from build123d import *

# Parameters (mm, degrees)
SKETCH1_R               = 12.7
SKETCH1_R_2             = 6.35
BOSS_EXTRUDE1_DEPTH     = 7.62
CUT_EXTRUDE1_DEPTH      = 7.619999999999999
CUT_EXTRUDE1_DEPTH_BACK = 10.16
BOSS_EXTRUDE2_DEPTH     = 7.619999999999999
SKETCH5_R               = 1.905
SKETCH5_R_2             = 1.9050000000000018
CUT_EXTRUDE2_DEPTH      = 7.619999999999999


with BuildPart() as part:
    # Sketch1 → Boss-Extrude1 (new body)
    # profile 1 of 2: a face of its own
    with BuildSketch(Plane.XY):
        with Locations((-11.43, -2.615954225782393)):
            Circle(SKETCH1_R)
        with Locations((-11.43, -2.615954225782393)):
            Circle(SKETCH1_R_2, mode=Mode.SUBTRACT)
    # profile 2 of 2: a face of its own
    with BuildSketch(Plane.XY):
        Polygon((-8.7e-16, 22.784045774217606), (0, -28.01595422578239), (3.175, -28.01595422578239), (3.174999999999999, 22.784045774217606), align=None)
    extrude(amount=BOSS_EXTRUDE1_DEPTH)

    # Sketch3 → Cut-Extrude1 (cut, two sides: drawn at the far end of the back side and taken through both)
    with BuildSketch(Plane(origin=(5.715, 1e-16, 0), x_dir=(0, 0, -1), z_dir=(1, 2e-17, 0)).offset(-CUT_EXTRUDE1_DEPTH_BACK)):
        with BuildLine():
            ThreePointArc((-1.905, 15.116671425817602), (-2.4629615818396333, 16.46370984397798), (-3.810000000000017, 17.0216714258176))
            Line((-3.81, 17.0216714258176), (-3.81, 15.116671425817602))
            Line((-3.81, 15.116671425817602), (-3.81, 13.211671425817602))
            ThreePointArc((-3.8100000000000174, 13.211671425817602), (-2.4629615818396333, 13.769633007657223), (-1.905, 15.116671425817602))
        make_face()
        with BuildLine():
            Line((-3.81, 15.116671425817602), (-3.81, 17.0216714258176))
            ThreePointArc((-3.810000000000017, 17.0216714258176), (-5.715, 15.116671425817602), (-3.8100000000000174, 13.211671425817602))
            Line((-3.81, 13.211671425817602), (-3.81, 15.116671425817602))
        make_face()
        with BuildLine():
            ThreePointArc((-1.9049999999999947, -20.395954225782393), (-2.4629615818396298, -19.048915807622013), (-3.810000000000017, -18.490954225782392))
            Line((-3.81, -18.490954225782392), (-3.81, -20.395954225782393))
            Line((-3.81, -20.395954225782393), (-3.81, -22.300954225782395))
            ThreePointArc((-3.8100000000000156, -22.300954225782395), (-2.462961581839629, -21.742992643942774), (-1.9049999999999947, -20.395954225782393))
        make_face()
        with BuildLine():
            Line((-3.81, -20.395954225782393), (-3.81, -18.490954225782392))
            ThreePointArc((-3.810000000000017, -18.490954225782392), (-5.7149999999999945, -20.395954225782393), (-3.8100000000000156, -22.300954225782395))
            Line((-3.81, -22.300954225782395), (-3.81, -20.395954225782393))
        make_face()
    extrude(amount=CUT_EXTRUDE1_DEPTH + CUT_EXTRUDE1_DEPTH_BACK, mode=Mode.SUBTRACT)

    # Sketch4 → Boss-Extrude2 (add)
    with BuildSketch(Plane.XY.offset(7.62)):
        Polygon((3.174999999999999, 22.784045774217606), (5.715, 22.784045774217606), (5.715000000000006, -27.992122779019148), (3.174999999999999, -27.992122779019148), align=None)
    extrude(amount=-BOSS_EXTRUDE2_DEPTH)

    # Sketch5 → Cut-Extrude2 (cut)
    with BuildSketch(Plane(origin=(5.7150000000000025, 6.8e-16, 0), x_dir=(0, 0, -1), z_dir=(1, 1.2e-16, 0))):
        with Locations(Location((-3.81, 15.116671425817602, 0), (0, 0, 270))):
            Circle(SKETCH5_R)
        with Locations(Location((-3.8099999999999947, -20.395954225782393, 0), (0, 0, 270))):
            Circle(SKETCH5_R_2)
    extrude(amount=-CUT_EXTRUDE2_DEPTH, mode=Mode.SUBTRACT)


solid = part.part
The model under review builds one solid part; all positions refer to its coordinate system, in mm. A direction names the side the tool comes from. Give positions to 0.01 mm unless a question says otherwise; leave off trailing zeros. Loops run counter-clockwise (first coordinate to the right, second up) from the corner with the lowest first, then second, coordinate; pieces in that order, holes last. Notation, with made-up numbers: (40, 29.25) -> (73, 29.25) arc R20 ccw to (73, 64.25) -> close; hole circle Ø6 at (-7, 13). An arc over 180 degrees is marked (long way). Put each result on its own line as item: value. Start each with the question number.
1. We need section C-C on y = 16. State the section outline as (x, z) points (3 decimals).
2. We need section B-B on z = 4.5. State the section outline as (x, y) points (3 decimals), then the cut area to 3 significant figures.
3. Wall thickness on probe 1 along Y at (x, z) = (1.45, 3.81); probe 2 along Y at (x, z) = (-11.43, 5); probe 3 along X at (y, z) = (-24, 1.5) (3 decimals): over which ranges is each line inside the solid? List them lowest first.
4. Clearance check with flat-ended pins moving along their axes: P1, Ø1.3, axis at x = 5, z = 3.5, coming from the -Y side; P2, Ø4.5, axis at y = 15.12, z = 3.81, coming from the +X side (3 decimals); P3, Ø4, axis at y = 11, z = 2.5, coming from the -X side. State where each tip first meets the part, or that it passes through.
5. We need section D-D on z = 6.75. State the section outline as (x, y) points (3 decimals), then the cut area to 3 significant figures.
6. For faces 1 (the face through (2, -28.016, 4)), 2 (the face through (0, 13, 4)), list the 3-axis set-ups (+Z, -Z, +X, -X, +Y, -Y) from which the entire face can be reached by the end or side of a thin tool; tool diameter is ignored.
7. Mouldability with a two-part tool opening along X and no side actions: class faces 3 (the face through (2.9, 16.5, 2.5)), 4 (the face through (5.715, -2, 4)), 5 (the face through (0, -18, 4)) as released by +X, released by -X, zero draft, split by the parting line, or undercut.
8. We need section A-A on x = -11.43. State the section outline as (y, z) points, then the cut area to 3 significant figures.
Determined:
1. outline: (0, 0) -> (5.715, 0) -> (5.715, 2.122) -> (0, 2.122) -> close; (0, 5.498) -> (5.715, 5.498) -> (5.715, 7.62) -> (0, 7.62) -> close
2. outline: (0, -28.016) -> (3.175, -28.016) -> (3.175, -27.992) -> (5.715, -27.992) -> (5.715, -22.172) -> (0, -22.172) -> close; (0, -18.62) -> (5.715, -18.62) -> (5.715, 13.341) -> (0, 13.341) -> (0, 2.92) arc R12.7 ccw (long way) to (0, -8.152) -> close; (0, 16.892) -> (5.715, 16.892) -> (5.715, 22.784) -> (0, 22.784) -> close; hole circle Ø12.7 at (-11.43, -2.616)
2. area: 620 mm^2
3. probe 1: -28.02 to -22.3, -18.49 to 13.21, 17.02 to 22.78
3. probe 2: -15.32 to -8.97, 3.73 to 10.08
3. probe 3: 0 to 5.715
4. P1: y = -27.99
4. P2: x = 5.715
4. P3: x = -16.56
5. outline: (0, -28.016) -> (3.175, -28.016) -> (3.175, -27.992) -> (5.715, -27.992) -> (5.715, 22.784) -> (0, 22.784) -> (0, 2.92) arc R12.7 ccw (long way) to (0, -8.152) -> close; hole circle Ø12.7 at (-11.43, -2.616)
5. area: 661 mm^2
6. face 1: +Z, -Z, +X, -X, -Y
6. face 2: +Z, -Z, +Y
7. face 3: zero draft
7. face 4: released by +X
7. face 5: undercut
8. outline: (-15.32, 0) -> (-8.97, 0) -> (-8.97, 7.62) -> (-15.32, 7.62) -> close; (3.73, 0) -> (10.08, 0) -> (10.08, 7.62) -> (3.73, 7.62) -> close
8. area: 96.8 mm^2
